Can you work these out from the model? Positions are in its coordinate system, mm. A direction names the side the tool comes from. Give positions to 0.01 mm unless a question says otherwise; leave off trailing zeros. Loops run counter-clockwise (first coordinate to the right, second up) from the corner with the lowest first, then second, coordinate; pieces in that order, holes last. Notation, with made-up numbers: (79.5, 80.25) - (97.5, 80.25) arc R28 ccw to (97.5, 107.25) - close; hole circle Ø3 at (72.25, -25.5). An arc over 180 degrees is marked (long way). Answer as a JSON object with one key per item and string values.
```python
from build123d import *

# Parameters (mm, degrees)
SKETCH_W        = 71
SKETCH_H        = 43
SKETCH_W_2      = 61
SKETCH_H_2      = 33
PAD_DEPTH       = 10
SKETCH001_W     = 5
SKETCH001_H     = 10
SKETCH001_W_2   = 10
SKETCH001_H_2   = 5
PAD001_DEPTH    = 120
SKETCH002_W     = 10
SKETCH002_H     = 5
PAD002_DEPTH    = 5
SKETCH003_W     = 16
SKETCH003_H     = 10
PAD003_DEPTH    = 5
CHAMFER_SIZE    = 5
SKETCH004_W     = 30
SKETCH004_H     = 30
SKETCH004_R     = 2.6
PAD004_DEPTH    = 5
CHAMFER001_SIZE = 5
CHAMFER002_SIZE = 2


with BuildPart() as part:
    # Sketch → Pad (new body)
    with BuildSketch(Plane.XY):
        Rectangle(SKETCH_W, SKETCH_H)
        Rectangle(SKETCH_W_2, SKETCH_H_2, mode=Mode.SUBTRACT)
    extrude(amount=PAD_DEPTH)

    # Sketch001 (on Face9 of Pad) → Pad001 (join)
    with BuildSketch(Plane(origin=(0, 0, 0), x_dir=(1, 0, 0), z_dir=(0, 0, -1))):
        with Locations((-33, 0)):
            Rectangle(SKETCH001_W, SKETCH001_H)
        with Locations((33, 0)):
            Rectangle(SKETCH001_W, SKETCH001_H)
        with Locations((0, -19)):
            Rectangle(SKETCH001_W_2, SKETCH001_H_2)
    extrude(amount=PAD001_DEPTH)

    # Sketch002 (on Face21 of Pad001) → Pad002 (join)
    with BuildSketch(Plane.XZ.offset(-16.5)):
        with Locations((0, -117.5)):
            Rectangle(SKETCH002_W, SKETCH002_H)
    extrude(amount=PAD002_DEPTH)

    # Sketch003 (on Face7 of Pad002) → Pad003 (join)
    with BuildSketch(Plane(origin=(0, 0, -120), x_dir=(1, 0, 0), z_dir=(0, 0, -1))):
        with Locations((-27.5, 0)):
            Rectangle(SKETCH003_W, SKETCH003_H)
        with Locations((27.5, 0)):
            Rectangle(SKETCH003_W, SKETCH003_H)
    extrude(amount=-PAD003_DEPTH)

    # Chamfer
    chamfer_edges = [part.edges().sort_by_distance(p)[0] for p in [
        (-5, 19, 0),
        (-33, 5, 0),
        (5, 19, 0),
        (33, 5, 0),
        (33, -5, 0),
        (-33, -5, 0),
        (35.5, 21.5, 5),
        (35.5, -21.5, 5),
        (-35.5, 21.5, 5),
        (-35.5, -21.5, 5),
    ]]
    chamfer(chamfer_edges, length=CHAMFER_SIZE)

    # Sketch004 (on Face13 of Chamfer) → Pad004 (join)
    with BuildSketch(Plane.XY.offset(10)):
        with Locations((0, 36.5)):
            Rectangle(SKETCH004_W, SKETCH004_H)
        with Locations((0, 36.5)):
            Circle(SKETCH004_R, mode=Mode.SUBTRACT)
    extrude(amount=-PAD004_DEPTH)

    # Chamfer001
    chamfer001_edges = [part.edges().sort_by_distance(p)[0] for p in [
        (15, 21.5, 7.5),
        (-15, 21.5, 7.5),
        (-15, 51.5, 7.5),
        (15, 51.5, 7.5),
    ]]
    chamfer(chamfer001_edges, length=CHAMFER001_SIZE)

    # Chamfer002
    chamfer002_edges = [part.edges().sort_by_distance(p)[0] for p in [
        (35.5, 0, -120),
        (0, 21.5, -120),
        (-35.5, 0, -120),
    ]]
    chamfer(chamfer002_edges, length=CHAMFER002_SIZE)


solid = part.part
```
1) I'm going to push flat-ended pins straight in: P1, Ø6, axis at x = -1, z = -105, coming from the +Y side; P2, Ø11, axis at y = 14.5, z = -65.5, coming from the -X side; P3, Ø1.5, axis at y = 36, z = 8, coming from the -X side; P4, Ø1.5, axis at y = 0, z = -118.5, coming from the -X side. Where does each tip first touch, or does it pass through?
Check sheet entries:
{"P1": "y = 21.5", "P2": "x = -5", "P3": "x = -15", "P4": "x = -35.5"}
2) Imagine slicing it at B-B on z = -73. Write out the boundary of the cut face in (x, y), and give its area (3 significant figures).
Check sheet entries:
{"outline": "(-35.5, -5) - (-30.5, -5) - (-30.5, 5) - (-35.5, 5) - close; (-5, 16.5) - (5, 16.5) - (5, 21.5) - (-5, 21.5) - close; (30.5, -5) - (35.5, -5) - (35.5, 5) - (30.5, 5) - close", "area": "150 mm2"}
3) I need wall thicknesses on L1, parallel to Y at x = 0, z = 8.6; L2, parallel to X at y = 0.5, z = -27.5; L3, parallel to Z at x = 27, y = -2.5. Which ranges of each line are inside material? Lowest first, please.
Check sheet entries:
{"L1": "-21.5 to -16.5, 16.5 to 33.9, 39.1 to 51.5", "L2": "-35.5 to -30.5, 30.5 to 35.5", "L3": "-120 to -115"}
4) If we mould it in two halves opening along X, with no side actions, what happens to faces 5 (the flat face through (-30.5, 0, -39)), 6 (the flat face through (5, 19, -63)), 7 (the flat face through (-12.5, 49, 7.5))? For each: released by +X, released by -X, zero draft, split by the parting line, or undercut.
Check sheet entries:
{"face 5": "undercut", "face 6": "released by +X", "face 7": "released by -X"}
5) Imagine slicing it at C-C on y = 36.5. Write out the boundary of the cut face in (x, z).
Check sheet entries:
{"outline": "(-15, 5) - (-2.6, 5) - (-2.6, 10) - (-15, 10) - close; (2.6, 5) - (15, 5) - (15, 10) - (2.6, 10) - close"}
6) Imagine slicing it at D-D on x = 8.5. Write out the boundary of the cut face in (y, z).
Check sheet entries:
{"outline": "(-21.5, 0) - (-16.5, 0) - (-16.5, 10) - (-21.5, 10) - close; (16.5, -1.5) - (21.5, -1.5) - (21.5, 5) - (51.5, 5) - (51.5, 10) - (16.5, 10) - close"}
7) Imagine slicing it at A-A on x = 0. Write out the boundary of the cut face in (y, z), and give its area (3 significant figures).
Check sheet entries:
{"outline": "(-21.5, 0) - (-16.5, 0) - (-16.5, 10) - (-21.5, 10) - close; (11.5, -120) - (19.5, -120) - (21.5, -118) - (21.5, 5) - (33.9, 5) - (33.9, 10) - (16.5, 10) - (16.5, -115) - (11.5, -115) - close; (39.1, 5) - (51.5, 5) - (51.5, 10) - (39.1, 10) - close", "area": "847 mm2"}
8) Which directions (+Z, -Z, +X, -X, +Y, -Y) give clear straight access to the entire face, cutting with the end or side of a thin tool? Please do faces 1 (the flat face through (15, 36, 8)), 2 (the flat face through (0, 51.5, 8)), 3 (the flat face through (-19.5, 0, -118)), 4 (the flat face through (33, -5, -66)).
Check sheet entries:
{"face 1": "+Z, -Z, +X, +Y", "face 2": "+Z, -Z, +X, -X, +Y", "face 3": "+Z, -Z, +Y, -Y", "face 4": "-Z, +X, -X, -Y"}
